from build123d import *

# Parameters (mm, degrees)
SKETCH1_R           = 1
BOSS_EXTRUDE1_DEPTH = 3


with BuildPart() as part:
    # Sketch1 → Boss-Extrude1 (new body)
    with BuildSketch(Plane.YZ):
        Polygon((-80, 60), (-80, 65), (-60, 65), (-60, 60), (-10, 60), (-10, 65), (10, 65), (10, 60), (60, 60), (60, 65), (80, 65), (80, 60), (100, 60), (100, -60), (80, -60), (80, -65), (60, -65), (60, -60), (10, -60), (10, -65), (-10, -65), (-10, -60), (-60, -60), (-60, -65), (-80, -65), (-80, -60), (-100, -60), (-100, 60), align=None)
        with Locations(Location((-5.445919919, 49.018671667, 0), (0, 0, 270))):
            Circle(SKETCH1_R, mode=Mode.SUBTRACT)
        with Locations(Location((4.554080081, 49.018671667, 0), (0, 0, 270))):
            Circle(SKETCH1_R, mode=Mode.SUBTRACT)
        with Locations(Location((14.554080081, 49.018671667, 0), (0, 0, 270))):
            Circle(SKETCH1_R, mode=Mode.SUBTRACT)
        with Locations(Location((24.554080081, 49.018671667, 0), (0, 0, 270))):
            Circle(SKETCH1_R, mode=Mode.SUBTRACT)
        with Locations(Location((34.554080081, 49.018671667, 0), (0, 0, 270))):
            Circle(SKETCH1_R, mode=Mode.SUBTRACT)
        with Locations(Location((44.554080081, 49.018671667, 0), (0, 0, 270))):
            Circle(SKETCH1_R, mode=Mode.SUBTRACT)
        with Locations(Location((54.554080081, 49.018671667, 0), (0, 0, 270))):
            Circle(SKETCH1_R, mode=Mode.SUBTRACT)
        with Locations(Location((64.554080081, 49.018671667, 0), (0, 0, 270))):
            Circle(SKETCH1_R, mode=Mode.SUBTRACT)
        with Locations(Location((-5.445919919, 29.018671667, 0), (0, 0, 270))):
            Circle(SKETCH1_R, mode=Mode.SUBTRACT)
        with Locations(Location((4.554080081, 29.018671667, 0), (0, 0, 270))):
            Circle(SKETCH1_R, mode=Mode.SUBTRACT)
        with Locations(Location((14.554080081, 29.018671667, 0), (0, 0, 270))):
            Circle(SKETCH1_R, mode=Mode.SUBTRACT)
        with Locations(Location((24.554080081, 29.018671667, 0), (0, 0, 270))):
            Circle(SKETCH1_R, mode=Mode.SUBTRACT)
        with Locations(Location((34.554080081, 29.018671667, 0), (0, 0, 270))):
            Circle(SKETCH1_R, mode=Mode.SUBTRACT)
        with Locations(Location((44.554080081, 29.018671667, 0), (0, 0, 270))):
            Circle(SKETCH1_R, mode=Mode.SUBTRACT)
        with Locations(Location((54.554080081, 29.018671667, 0), (0, 0, 270))):
            Circle(SKETCH1_R, mode=Mode.SUBTRACT)
        with Locations(Location((64.554080081, 29.018671667, 0), (0, 0, 270))):
            Circle(SKETCH1_R, mode=Mode.SUBTRACT)
        with Locations(Location((-5.445919919, 9.018671667, 0), (0, 0, 270))):
            Circle(SKETCH1_R, mode=Mode.SUBTRACT)
        with Locations(Location((4.554080081, 9.018671667, 0), (0, 0, 270))):
            Circle(SKETCH1_R, mode=Mode.SUBTRACT)
        with Locations(Location((14.554080081, 9.018671667, 0), (0, 0, 270))):
            Circle(SKETCH1_R, mode=Mode.SUBTRACT)
        with Locations(Location((24.554080081, 9.018671667, 0), (0, 0, 270))):
            Circle(SKETCH1_R, mode=Mode.SUBTRACT)
        with Locations(Location((34.554080081, 9.018671667, 0), (0, 0, 270))):
            Circle(SKETCH1_R, mode=Mode.SUBTRACT)
        with Locations(Location((44.554080081, 9.018671667, 0), (0, 0, 270))):
            Circle(SKETCH1_R, mode=Mode.SUBTRACT)
        with Locations(Location((54.554080081, 9.018671667, 0), (0, 0, 270))):
            Circle(SKETCH1_R, mode=Mode.SUBTRACT)
        with Locations(Location((64.554080081, 9.018671667, 0), (0, 0, 270))):
            Circle(SKETCH1_R, mode=Mode.SUBTRACT)
        with Locations(Location((-5.445919919, -10.981328333, 0), (0, 0, 270))):
            Circle(SKETCH1_R, mode=Mode.SUBTRACT)
        with Locations(Location((4.554080081, -10.981328333, 0), (0, 0, 270))):
            Circle(SKETCH1_R, mode=Mode.SUBTRACT)
        with Locations(Location((14.554080081, -10.981328333, 0), (0, 0, 270))):
            Circle(SKETCH1_R, mode=Mode.SUBTRACT)
        with Locations(Location((24.554080081, -10.981328333, 0), (0, 0, 270))):
            Circle(SKETCH1_R, mode=Mode.SUBTRACT)
        with Locations(Location((34.554080081, -10.981328333, 0), (0, 0, 270))):
            Circle(SKETCH1_R, mode=Mode.SUBTRACT)
        with Locations(Location((44.554080081, -10.981328333, 0), (0, 0, 270))):
            Circle(SKETCH1_R, mode=Mode.SUBTRACT)
        with Locations(Location((54.554080081, -10.981328333, 0), (0, 0, 270))):
            Circle(SKETCH1_R, mode=Mode.SUBTRACT)
        with Locations(Location((64.554080081, -10.981328333, 0), (0, 0, 270))):
            Circle(SKETCH1_R, mode=Mode.SUBTRACT)
        with Locations(Location((-5.445919919, -30.981328333, 0), (0, 0, 270))):
            Circle(SKETCH1_R, mode=Mode.SUBTRACT)
        with Locations(Location((4.554080081, -30.981328333, 0), (0, 0, 270))):
            Circle(SKETCH1_R, mode=Mode.SUBTRACT)
        with Locations(Location((14.554080081, -30.981328333, 0), (0, 0, 270))):
            Circle(SKETCH1_R, mode=Mode.SUBTRACT)
        with Locations(Location((24.554080081, -30.981328333, 0), (0, 0, 270))):
            Circle(SKETCH1_R, mode=Mode.SUBTRACT)
        with Locations(Location((34.554080081, -30.981328333, 0), (0, 0, 270))):
            Circle(SKETCH1_R, mode=Mode.SUBTRACT)
        with Locations(Location((44.554080081, -30.981328333, 0), (0, 0, 270))):
            Circle(SKETCH1_R, mode=Mode.SUBTRACT)
        with Locations(Location((54.554080081, -30.981328333, 0), (0, 0, 270))):
            Circle(SKETCH1_R, mode=Mode.SUBTRACT)
        with Locations(Location((64.554080081, -30.981328333, 0), (0, 0, 270))):
            Circle(SKETCH1_R, mode=Mode.SUBTRACT)
        with Locations(Location((-5.445919919, -50.981328333, 0), (0, 0, 270))):
            Circle(SKETCH1_R, mode=Mode.SUBTRACT)
        with Locations(Location((4.554080081, -50.981328333, 0), (0, 0, 270))):
            Circle(SKETCH1_R, mode=Mode.SUBTRACT)
        with Locations(Location((14.554080081, -50.981328333, 0), (0, 0, 270))):
            Circle(SKETCH1_R, mode=Mode.SUBTRACT)
        with Locations(Location((24.554080081, -50.981328333, 0), (0, 0, 270))):
            Circle(SKETCH1_R, mode=Mode.SUBTRACT)
        with Locations(Location((34.554080081, -50.981328333, 0), (0, 0, 270))):
            Circle(SKETCH1_R, mode=Mode.SUBTRACT)
        with Locations(Location((44.554080081, -50.981328333, 0), (0, 0, 270))):
            Circle(SKETCH1_R, mode=Mode.SUBTRACT)
        with Locations(Location((54.554080081, -50.981328333, 0), (0, 0, 270))):
            Circle(SKETCH1_R, mode=Mode.SUBTRACT)
        with Locations(Location((64.554080081, -50.981328333, 0), (0, 0, 270))):
            Circle(SKETCH1_R, mode=Mode.SUBTRACT)
        with Locations(Location((-70, 61, 0), (0, 0, 270))):
            Circle(SKETCH1_R, mode=Mode.SUBTRACT)
        with Locations(Location((70, 61, 0), (0, 0, 270))):
            Circle(SKETCH1_R, mode=Mode.SUBTRACT)
        with Locations(Location((0, 61, 0), (0, 0, 270))):
            Circle(SKETCH1_R, mode=Mode.SUBTRACT)
        with Locations(Location((70, -61, 0), (0, 0, 270))):
            Circle(SKETCH1_R, mode=Mode.SUBTRACT)
        with Locations(Location((0, -61, 0), (0, 0, 270))):
            Circle(SKETCH1_R, mode=Mode.SUBTRACT)
        with Locations(Location((-70, -61, 0), (0, 0, 270))):
            Circle(SKETCH1_R, mode=Mode.SUBTRACT)
    extrude(amount=BOSS_EXTRUDE1_DEPTH)


solid = part.part
Verification items for the finished model (mm, model axes). Coordinates: 2 decimals unless noted, no trailing zeros. Loops run counter-clockwise (first coordinate to the right, second up) from the corner with the lowest first, then second, coordinate; pieces in that order, holes last. Notation, with made-up numbers: (-2.75, 22.25) -> (24.25, 22.25) arc R20 ccw to (24.25, 61.25) -> close; hole circle Ø1 at (71, 26). An arc over 180 degrees is marked (long way). Write each question's results on one line, items separated by ' | '.
Item 1: Material ranges on L1, parallel to Y at x = 2.3, z = 61; L2, parallel to Z at x = 1.1, y = -70; L3, parallel to Z at x = 0.85, y = -16, recorded low to high.
Found:
L1: y = -80 to -71, -69 to -60, -10 to -1, 1 to 10, 60 to 69, 71 to 80 | L2: z = -65 to -62, -60 to 60, 62 to 65 | L3: z = -60 to 60
Item 2: Section check B-B, the plane x = 0.6. Count the separate pieces of the cut face and the enclosed holes in it, plus the area to 3 significant figures.
Found:
separate pieces: 1 | enclosed holes: 54 | area: 24,400 mm2
Item 3: Section check A-A, the plane y = -44.5. Enter the section's corners in (x, z), plus the area to 3 significant figures.
Found:
outline: (0, -60) -> (3, -60) -> (3, 60) -> (0, 60) -> close | area: 360 mm2
Item 4: Gauge pin test, flat ends, axial feed: pin 1 (0.9 mm diameter, centred on x = 2, z = 62, fed in from +Y); pin 2 (1.8 mm diameter, centred on y = 54.55, z = 29.02, fed in from -X); pin 3 (1 mm diameter, centred on x = 2, y = -55.5, fed in from +Z). Record the tip position at first contact, or that the pin passes through.
Found:
pin 1: stops at y = 80 | pin 2: passes through | pin 3: stops at z = 60
